The listing builds one solid part. Answer for the finished solid, in the listing's coordinates (mm). A direction names the side the tool comes from. Coordinates: 2 decimals unless noted, no trailing zeros. Order: outer loops, then holes, each group sorted by start corner. A loop starts at its lowest first (then second) coordinate and runs counter-clockwise, first axis right, second up. Notation, with made-up numbers: (-19.75, -33) -> (-9.75, -33) arc R27 cw to (-9.75, -8) -> close; hole circle Ø2 at (25, 78). An arc over 180 degrees is marked (long way). Return JSON: item names as keys, results as strings.
```python
from build123d import *

# Parameters (mm, degrees)
F0_W     = 88.9
F0_H     = 50.8
F1_DEPTH = 76.2
F2_R     = 16.335339
F3_DEPTH = 19.05
F4_W     = 4.892699
F4_H     = 4.604891
F4_W_2   = 4.317085
F4_H_2   = 4.029282
F5_DEPTH = 12.7
F6_W     = 6.043921
F6_H     = 4.892695
F6_W_2   = 5.180505
F6_H_2   = 5.1805
F7_DEPTH = 6.35


with BuildPart() as f1:
    # F0 (on Top) → F1 (new body)
    with BuildSketch(Plane.XY):
        with Locations((-4.012393, -24.22007)):
            Rectangle(F0_W, F0_H)
    extrude(amount=F1_DEPTH)

    # F2 (on Top) → F3 (cut)
    with BuildSketch(Plane.XY):
        with Locations((-4.748795, -26.145704)):
            Circle(F2_R)
    extrude(amount=F3_DEPTH, mode=Mode.SUBTRACT)

    # F4 (on Top) → F5 (join)
    with BuildSketch(Plane.XY):
        with Locations((-21.873237, -44.178185)):
            Rectangle(F4_W, F4_H)
        with Locations((9.785395, -44.178184)):
            Rectangle(F4_W_2, F4_H_2)
    extrude(amount=F5_DEPTH)

    # F6 (on Top) → F7 (join)
    with BuildSketch(Plane.XY):
        with Locations((-19.282984, -44.322086)):
            Rectangle(F6_W, F6_H)
        with Locations((7.914659, -44.465989)):
            Rectangle(F6_W_2, F6_H_2)
    extrude(amount=-F7_DEPTH)


solid = f1.part
```
Item 1: The part is cut by section B-B on z = 12.5. Determine the outline of the cut face in (x, y).
Answer list:
{"outline": "(-48.46, -49.62) -> (40.44, -49.62) -> (40.44, 1.18) -> (-48.46, 1.18) -> close; hole circle Ø32.67 at (-4.75, -26.15)"}
Item 2: The part is cut by section C-C on x = -10. Determine the outline of the cut face in (y, z), plus the area to 3 significant figures.
Answer list:
{"outline": "(-49.62, 0) -> (-41.61, 0) -> (-41.61, 19.05) -> (-10.68, 19.05) -> (-10.68, 0) -> (1.18, 0) -> (1.18, 76.2) -> (-49.62, 76.2) -> close", "area": "3,280 mm2"}
Item 3: Determine the mould class of faces 1 (the flat face through (8, -41.876, -3)), 2 (the flat face through (40.438, -25, 38)), 3 (the flat face through (-16.261, -44, -3)) for opening direction X: pulls with the +X half, pulls with the -X half, needs draft (parallel to the pull), parting line crosses it, or undercut.
Answer list:
{"face 1": "needs draft", "face 2": "pulls with the +X half", "face 3": "undercut"}
Item 4: The part is cut by section D-D on y = -35. Determine the outline of the cut face in (x, z).
Answer list:
{"outline": "(-48.46, 0) -> (-18.48, 0) -> (-18.48, 19.05) -> (8.98, 19.05) -> (8.98, 0) -> (40.44, 0) -> (40.44, 76.2) -> (-48.46, 76.2) -> close"}
Item 5: Find the intervals of material crossed by probe 1 along Z at (x, y) = (-1, -39.5); probe 2 along Z at (x, y) = (-13, -8); probe 3 along X at (y, z) = (-30, 14), in increasing order.
Answer list:
{"probe 1": "19.05 to 76.2", "probe 2": "0 to 76.2", "probe 3": "-48.46 to -20.62, 11.13 to 40.44"}
Item 6: The part is cut by section A-A on y = -45. Determine the outline of the cut face in (x, z).
Answer list:
{"outline": "(-48.46, 0) -> (-22.3, 0) -> (-22.3, -6.35) -> (-16.26, -6.35) -> (-16.26, 0) -> (5.32, 0) -> (5.32, -6.35) -> (10.5, -6.35) -> (10.5, 0) -> (40.44, 0) -> (40.44, 76.2) -> (-48.46, 76.2) -> close"}
Item 7: Flat-ended cylindrical pins translate along their axes: pin 1 (16.5 mm diameter, centred on x = 0.5, y = -29.5, fed in from -Z); pin 2 (4 mm diameter, centred on x = -21.5, y = -15, fed in from -Z); pin 3 (2.5 mm diameter, centred on x = 8.5, z = -2, fed in from +Y). Find the tip coordinate at first contact, or state that the pin passes through.
Answer list:
{"pin 1": "z = 19.05", "pin 2": "z = 0", "pin 3": "y = -41.88"}
Item 8: Which of the six approach directions +Z, -Z, +X, -X, +Y, -Y give full straight-line access (tool end or side, diameter ignored) to faces 4 (the flat face through (-19, -46.768, -3)), 5 (the flat face through (8, -47.056, -3)), 6 (the cylindrical face through (-8.29, -42.093, 9.392))?
Answer list:
{"face 4": "-Z, -X, -Y", "face 5": "-Z, +X, -X, -Y", "face 6": "-Z"}
